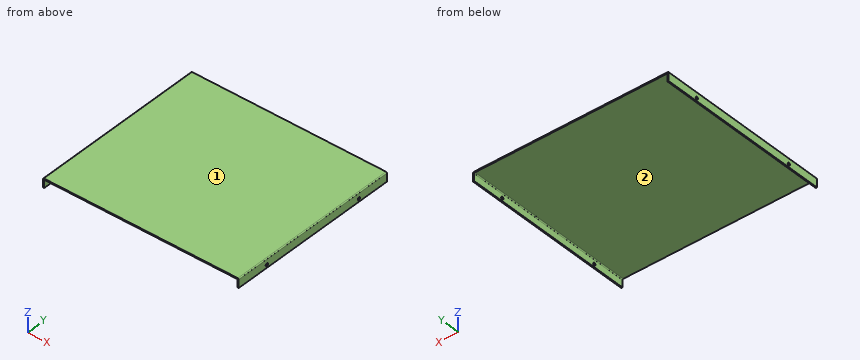
```python
from build123d import *

# Parameters (mm, degrees)
ESQUISSE1_W           = 320
ESQUISSE1_H           = 290
BOSS_EXTRU_1_DEPTH    = 2
ESQUISSE2_W           = 15
ESQUISSE2_H           = 290
BOSS_EXTRU_2_DEPTH    = 2
CONG_1_R              = 1.5
CONG_1_OF_SYM_TRIE1_R = 1.5
D_GAGEMENT_M41_D      = 4.5


with BuildPart() as part:
    # Esquisse1 → Boss.-Extru.1 (new body)
    with BuildSketch(Plane.XY):
        Rectangle(ESQUISSE1_W, ESQUISSE1_H)
    extrude(amount=BOSS_EXTRU_1_DEPTH)

    # Esquisse2 → Boss.-Extru.2 (add)
    with BuildSketch(Plane.ZY.offset(160)):
        with Locations((-5.5, 0)):
            Rectangle(ESQUISSE2_W, ESQUISSE2_H)
    boss_extru_2 = extrude(amount=BOSS_EXTRU_2_DEPTH)

    # Congé1
    cong_1_edges = [part.edges().sort_by_distance(p)[0] for p in [
        (-160, 0, 0),
        (-162, 0, 2),
    ]]
    fillet(cong_1_edges, radius=CONG_1_R)

    # Symétrie1: Boss.-Extru.2 across plane
    add(boss_extru_2.mirror(Plane(origin=(0, 0, 0), x_dir=(0, 0, 1), z_dir=(1, 0, 0))))

    # Congé1 of Symétrie1
    cong_1_of_sym_trie1_edges = [part.edges().sort_by_distance(p)[0] for p in [
        (160, 0, 0),
        (162, 0, 2),
    ]]
    fillet(cong_1_of_sym_trie1_edges, radius=CONG_1_OF_SYM_TRIE1_R)

    # Dégagement M41 (through all)
    with Locations(Plane.ZY.offset(162)):
        with Locations((-8, -90), (-8, 90)):
            Hole(D_GAGEMENT_M41_D / 2)


solid = part.part
```
Geometry: final body of the model. Coordinates: model frame, mm. Face numbers are marked on the shaded views. Coordinates: 2 decimals unless noted, no trailing zeros. Loops run counter-clockwise (first coordinate to the right, second up) from the corner with the lowest first, then second, coordinate; pieces in that order, holes last. Notation, with made-up numbers: (27.25, 41) -> (42.25, 41) arc R27 cw to (42.25, 65) -> close; hole circle Ø5 at (-25.5, -14.75). An arc over 180 degrees is marked (long way). Use a Markdown table: item, result. Add a question column.
(1) Section query A-A, the plane z = -8. Return loops of the section in (x, y).
(2) Section query C-C, the plane x = 52.5. Return loops of the section in (y, z), plus the area to 3 significant figures.
(3) Section query B-B, the plane y = -67.5. Return loops of the section in (x, z).
(4) Pin query (flat end, axial travel): pin 1 Ø8 at (x, y) = (-121.5, -97.5) entering from -Z. Return the tip coordinate at first contact, or that it passes through.
(5) Mould query, pull axis X, two halves, no side actions, for the marked faces 1 and 2. Classes: pulls with the +X half, pulls with the -X half, needs draft (parallel to the pull), parting line crosses it, or undercut.
(6) Line query: line 1 along Y through (x, z) = (160.8, -8); line 2 along X through (y, z) = (54, -12.5); line 3 along Z through (x, y) = (-57.5, 96). Output: solid intervals per line, ascending.
Answer:
| question | item | result |
|---|---|---|
| 1 | outline | (-162, -145) -> (-160, -145) -> (-160, -92.25) -> (-162, -92.25) -> close; (-162, -87.75) -> (-160, -87.75) -> (-160, 87.75) -> (-162, 87.75) -> close; (-162, 92.25) -> (-160, 92.25) -> (-160, 145) -> (-162, 145) -> close; (160, -145) -> (162, -145) -> (162, -92.25) -> (160, -92.25) -> close; (160, -87.75) -> (162, -87.75) -> (162, 87.75) -> (160, 87.75) -> close; (160, 92.25) -> (162, 92.25) -> (162, 145) -> (160, 145) -> close |
| 2 | outline | (-145, 0) -> (145, 0) -> (145, 2) -> (-145, 2) -> close |
| 2 | area | 580 mm^2 |
| 3 | outline | (-162, -13) -> (-160, -13) -> (-160, -1.5) arc R1.5 cw to (-158.5, 0) -> (158.5, 0) arc R1.5 cw to (160, -1.5) -> (160, -13) -> (162, -13) -> (162, 0.5) arc R1.5 ccw to (160.5, 2) -> (-160.5, 2) arc R1.5 ccw to (-162, 0.5) -> close |
| 4 | pin 1 | stops at z = 0 |
| 5 | face 1 | needs draft |
| 5 | face 2 | undercut |
| 6 | line 1 | y = -145 to -92.25, -87.75 to 87.75, 92.25 to 145 |
| 6 | line 2 | x = -162 to -160, 160 to 162 |
| 6 | line 3 | z = 0 to 2 |
